Part model, mm, in its own coordinate system. Face numbers are marked on the shaded views. A direction names the side the tool comes from. Give positions to 0.01 mm unless a question says otherwise; leave off trailing zeros. Loops run counter-clockwise (first coordinate to the right, second up) from the corner with the lowest first, then second, coordinate; pieces in that order, holes last. Notation, with made-up numbers: M 30,56.25 L 49,56.25 A18 cw 49,61.25 Z; hole C 41.25,27 d7. An arc over 180 degrees is marked long. Put each result on its own line as item: value. Start each with the question number.
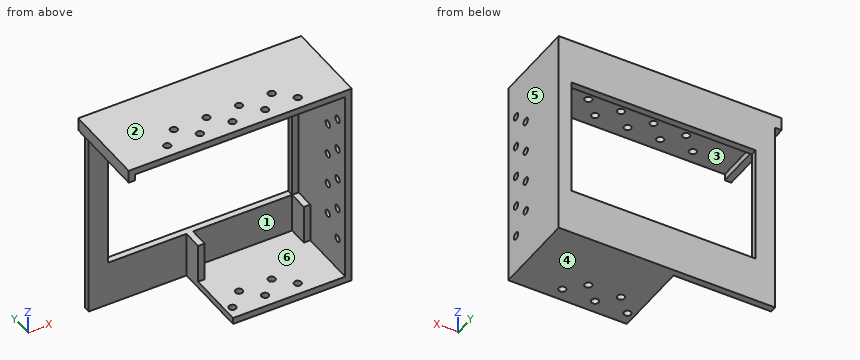
```python
from build123d import *

# Parameters (mm, degrees)
SKETCH1_W                      = 170.999999046
SKETCH1_H                      = 160.999999046
BOSS_EXTRUDE1_DEPTH            = 5
SKETCH2_W                      = 150.999999046
SKETCH2_H                      = 5
CUT_EXTRUDE1_DEPTH             = 5
SKETCH3_W                      = 140.999999046
SKETCH3_H                      = 5
CUT_EXTRUDE2_DEPTH             = 91.000001431
BOSS_EXTRUDE2_DEPTH            = 60
SKETCH5_W                      = 30
SKETCH5_H                      = 45
CUT_EXTRUDE3_DEPTH             = 81.000001431
CUT_EXTRUDE4_REACH             = 159.636
SKETCH7_W                      = 76.000001431
SKETCH7_H                      = 30
SKETCH8_W                      = 115.999999046
SKETCH8_H                      = 60
CUT_EXTRUDE5_DEPTH             = 5
SKETCH9_W                      = 5
SKETCH9_H                      = 30
CUT_EXTRUDE6_DEPTH             = 45
CUT_EXTRUDE7_REACH             = 197.582
SKETCH10_W                     = 155.999999046
SKETCH10_H                     = 60
SKETCH11_W                     = 5
SKETCH11_H                     = 45
CUT_EXTRUDE8_DEPTH             = 5
F_5_5_5_5_DIAMETER_HOLE1_D     = 5.5
F_5_5_5_5_DIAMETER_HOLE2_D     = 5.5
F_5_5_5_5_DIAMETER_HOLE2_DEPTH = 5
F_5_5_5_5_DIAMETER_HOLE3_D     = 5.5
RIB1_START                     = -2.5
RIB1_OUTLINE_W                 = 10
RIB1_OUTLINE_H                 = 15
RIB1_DEPTH                     = 5


# Read off the part's stored shape, not the designer's step: Rib1
with BuildPart() as part:
    # Sketch1 → Boss-Extrude1 (new body)
    with BuildSketch(Plane.XZ):
        with Locations((16.069853306, -24.060089588)):
            Rectangle(SKETCH1_W, SKETCH1_H)
    extrude(amount=-BOSS_EXTRUDE1_DEPTH)

    # Sketch2 → Cut-Extrude1 (cut)
    with BuildSketch(Plane.ZY.offset(69.430146217)):
        with Locations((-29.060089588, 2.5)):
            Rectangle(SKETCH2_W, SKETCH2_H)
    extrude(amount=-CUT_EXTRUDE1_DEPTH, mode=Mode.SUBTRACT)

    # Sketch3 → Cut-Extrude2 (cut)
    with BuildSketch(Plane(origin=(0, 0, -69.560089111), x_dir=(-1, 0, 0), z_dir=(0, 0, -1))):
        with Locations((-21.069853306, 2.5)):
            Rectangle(SKETCH3_W, SKETCH3_H)
    extrude(amount=-CUT_EXTRUDE2_DEPTH, mode=Mode.SUBTRACT)

    # Sketch4 → Boss-Extrude2 (add)
    with BuildSketch(Plane.XZ):
        Polygon((91.569852829, 46.439909935), (-69.430146217, 46.439909935), (-69.430146217, 56.439909935), (101.569852829, 56.439909935), (101.569852829, -104.560089111), (10.569851398, -104.560089111), (10.569851398, -69.560089111), (91.569852829, -69.560089111), align=None)
    extrude(amount=BOSS_EXTRUDE2_DEPTH)

    # Sketch5 → Cut-Extrude3 (cut)
    with BuildSketch(Plane.ZY.offset(-10.569851398)):
        with Locations((-84.560089111, -37.5)):
            Rectangle(SKETCH5_W, SKETCH5_H)
    extrude(amount=-CUT_EXTRUDE3_DEPTH, mode=Mode.SUBTRACT)

    # Sketch7 → Cut-Extrude4 (cut, up to next)
    with BuildSketch(Plane(origin=(0, 0, 0), x_dir=(1, 0, 0), z_dir=(0, 1, 0)), mode=Mode.PRIVATE) as cut_extrude4_sk1:
        with Locations((53.569852114, 84.560089111)):
            Rectangle(SKETCH7_W, SKETCH7_H)
    cut_extrude4_tool1 = extrude(cut_extrude4_sk1.sketch, amount=-CUT_EXTRUDE4_REACH, mode=Mode.PRIVATE) & part.part
    add(cut_extrude4_tool1.solids().sort_by_distance((53.569852, 0, -84.560089))[0], mode=Mode.SUBTRACT)

    # Sketch8 → Cut-Extrude5 (cut)
    with BuildSketch(Plane.ZY.offset(-91.569852829)):
        with Locations((-11.560089588, -30)):
            Rectangle(SKETCH8_W, SKETCH8_H)
    extrude(amount=-CUT_EXTRUDE5_DEPTH, mode=Mode.SUBTRACT)

    # Sketch9 → Cut-Extrude6 (cut)
    with BuildSketch(Plane.XZ.offset(60)):
        with Locations((94.069852829, -84.560089111)):
            Rectangle(SKETCH9_W, SKETCH9_H)
    extrude(amount=-CUT_EXTRUDE6_DEPTH, mode=Mode.SUBTRACT)

    # Sketch10 → Cut-Extrude7 (cut, up to next)
    with BuildSketch(Plane.XY.offset(51.439909935), mode=Mode.PRIVATE) as cut_extrude7_sk1:
        with Locations((18.569853306, -30)):
            Rectangle(SKETCH10_W, SKETCH10_H)
    cut_extrude7_tool1 = extrude(cut_extrude7_sk1.sketch, amount=-CUT_EXTRUDE7_REACH, mode=Mode.PRIVATE) & part.part
    add(cut_extrude7_tool1.solids().sort_by_distance((18.569853, -30, 51.43991))[0], mode=Mode.SUBTRACT)

    # Sketch11 → Cut-Extrude8 (cut)
    with BuildSketch(Plane(origin=(0, 0, 46.439909935), x_dir=(-1, 0, 0), z_dir=(0, 0, -1))):
        with Locations((61.930146217, -37.5)):
            Rectangle(SKETCH11_W, SKETCH11_H)
    extrude(amount=-CUT_EXTRUDE8_DEPTH, mode=Mode.SUBTRACT)

    # Ø5.5 (5.5) Diameter Hole1 (through all)
    with Locations(Plane.ZY.offset(-96.569852829)):
        with Locations((-61.560090383, -37.500000596), (-74.06009078, -50.000000795), (-49.059914748, -50.000000795), (-36.560089588, -37.500000596), (-11.560088396, -37.500000596), (13.439912299, -37.500000596), (0.939911927, -50.000000795), (25.939911604, -50.000000795), (-24.060088595, -50.000000795)):
            Hole(F_5_5_5_5_DIAMETER_HOLE1_D / 2)

    # Ø5.5 (5.5) Diameter Hole2
    with Locations(Plane(origin=(0, 0, 51.439909935), x_dir=(-1, 0, 0), z_dir=(0, 0, -1))):
        with Locations((33.93014888, -50.000000795), (21.430148681, -37.500000596), (8.93014883, -50.000000795), (-3.569851859, -37.500000596), (-16.069851716, -50.000000795), (-28.569851518, -37.500000596), (-41.069852312, -50.000000795), (-53.569852511, -37.500000596), (-66.069851716, -50.000000795)):
            Hole(F_5_5_5_5_DIAMETER_HOLE2_D / 2, depth=F_5_5_5_5_DIAMETER_HOLE2_DEPTH)

    # Ø5.5 (5.5) Diameter Hole3 (through all)
    with Locations(Plane.XY.offset(-99.560089111)):
        with Locations((16.069851716, -50.000000795), (28.569851518, -37.500000596), (41.069852312, -50.000000795), (53.569852511, -37.500000596), (66.069851716, -50.000000795)):
            Hole(F_5_5_5_5_DIAMETER_HOLE3_D / 2)

    # Rib1 outline → Rib1 (add)
    with BuildSketch(Plane(origin=(18.069851398, 0, 0), x_dir=(0, 0, -1), z_dir=(1, 0, 0)).offset(RIB1_START)):
        with Locations((-46.439909935, -7.5)):
            Rectangle(RIB1_OUTLINE_W, RIB1_OUTLINE_H)
    extrude(amount=RIB1_DEPTH)


solid = part.part
```
1) Band-saw the part on A-A on x = 88.5. Give the cut face in (y, z).
2) Which spindle directions (+Z, -Z, +X, -X, +Y, -Y) get a long thin tool onto all of the face, cutting with end or side? Do the marked faces 1 and 2. Say none if no direction does.
3) Pin check, flat tips, straight feed: pin 1 Ø5 at (x, y) = (-63.5, -27.5) entering from -Z; pin 2 Ø7 at (y, z) = (-50, -24.06) entering from +X; pin 3 Ø18 at (y, z) = (-34.5, 1.5) entering from -X. Stop position of each tip, or through.
4) Band-saw the part on C-C on z = -61. Give the cut face in (x, y).
5) Wall check: L1, parallel to X at y = -37.5, z = -102.15; L2, parallel to X at y = -37.5, z = 53.7; L3, parallel to Z at x = 98, y = -37. Give the ranges that are in metal, low to high.
6) Band-saw the part on D-D on y = -37.5. State how many separate pieces and enclosed holes the cut face has, then the cut area to 4 significant figures.
7) Mould opens along X. For the marked faces 3, 4, 5 and 6 say: +X half, -X half, draft (parallel to the pull), parting line (faces both ways), or undercut.
8) Band-saw the part on B-B on y = -22. Give the cut face in (x, z), then the cut area to 3 significant figures.
Evaluation:
1. outline: M -60,-104.56 L 5,-104.56 L 5,-69.56 L 0,-69.56 L 0,-99.56 L -60,-99.56 Z; M -60,51.44 L 0,51.44 L 0,21.44 L 5,21.44 L 5,56.44 L -60,56.44 Z
2. face 1: -Y
2. face 2: +Z, +X, -X, +Y, -Y
3. pin 1: z = 46.44
3. pin 2: x = 101.57
3. pin 3: x = 96.57
4. outline: M -64.43,0 L -49.43,0 L -49.43,5 L -64.43,5 Z; M 91.57,0 L 96.57,0 L 96.57,-34.81 L 101.57,-34.81 L 101.57,5 L 91.57,5 Z; M 96.57,-60 L 101.57,-60 L 101.57,-40.19 L 96.57,-40.19 Z
5. L1: 10.57 to 25.82, 31.32 to 50.82, 56.32 to 101.57
5. L2: -69.43 to -24.18, -18.68 to 0.82, 6.32 to 25.82, 31.32 to 50.82, 56.32 to 101.57
5. L3: -104.56 to -64.26, -58.86 to -39.26, -33.86 to -14.26, -8.86 to 10.74, 16.14 to 56.44
6. separate pieces: 11
6. enclosed holes: 0
6. area: 1,815 mm2
7. face 3: undercut
7. face 4: draft
7. face 5: +X half
7. face 6: undercut
8. outline: M -69.43,46.44 L -64.43,46.44 L -64.43,51.44 L 96.57,51.44 L 96.57,-99.56 L 10.57,-99.56 L 10.57,-104.56 L 101.57,-104.56 L 101.57,56.44 L -69.43,56.44 Z
8. area: 2,090 mm2
